For this review, take the finished solid that the model builds, in its own axes (mm). Round coordinates to 2 decimals unless told otherwise and drop trailing zeros. Order: outer loops, then holes, each group sorted by start corner. A loop starts at its lowest first (then second) coordinate and runs counter-clockwise, first axis right, second up. Notation, with made-up numbers: (70, 29.5) - (93, 29.5) arc R27 ccw to (93, 48.5) - close; hole circle Ø9 at (-26, -15). An arc over 180 degrees is marked (long way). One line per item, written item: value.
```python
from build123d import *

# Parameters (mm, degrees)
SKETCH1_W                                           = 50.8
SKETCH1_H                                           = 381
BASE_EXTRUDE_DEPTH                                  = 12.7
CSK_FOR_1_4_FLAT_HEAD_MACHINE_SCREW_100_D           = 6.7564
CSK_FOR_1_4_FLAT_HEAD_MACHINE_SCREW_100_CSINK_D     = 12.8778
CSK_FOR_1_4_FLAT_HEAD_MACHINE_SCREW_100_CSINK_ANGLE = 100
FILLET1_R                                           = 6.35
FILLET2_R                                           = 3.048


with BuildPart() as part:
    # Sketch1 → Base-Extrude (new body)
    with BuildSketch(Plane.XY):
        Rectangle(SKETCH1_W, SKETCH1_H)
    extrude(amount=BASE_EXTRUDE_DEPTH)

    # CSK for 1/4 Flat Head Machine Screw (100)1 (through all)
    with Locations(Plane.XY.offset(12.7)):
        with Locations((0, 165.1), (0, -165.1)):
            CounterSinkHole(CSK_FOR_1_4_FLAT_HEAD_MACHINE_SCREW_100_D / 2, CSK_FOR_1_4_FLAT_HEAD_MACHINE_SCREW_100_CSINK_D / 2, counter_sink_angle=CSK_FOR_1_4_FLAT_HEAD_MACHINE_SCREW_100_CSINK_ANGLE)

    # Fillet1
    fillet1_edges = [part.edges().sort_by_distance(p)[0] for p in [
        (25.4, -190.5, 6.35),
        (-25.4, -190.5, 6.35),
        (-25.4, 190.5, 6.35),
        (25.4, 190.5, 6.35),
    ]]
    fillet(fillet1_edges, radius=FILLET1_R)

    # Fillet2
    fillet2_edges = [part.edges().sort_by_distance(p)[0] for p in [
        (25.4, 0, 12.7),
        (0, -190.5, 12.7),
        (0, 190.5, 12.7),
        (-25.4, 0, 12.7),
        (23.540128061, 188.640128061, 12.7),
        (-23.540128061, 188.640128061, 12.7),
        (-23.540128061, -188.640128061, 12.7),
        (23.540128061, -188.640128061, 12.7),
    ]]
    fillet(fillet2_edges, radius=FILLET2_R)


solid = part.part
```
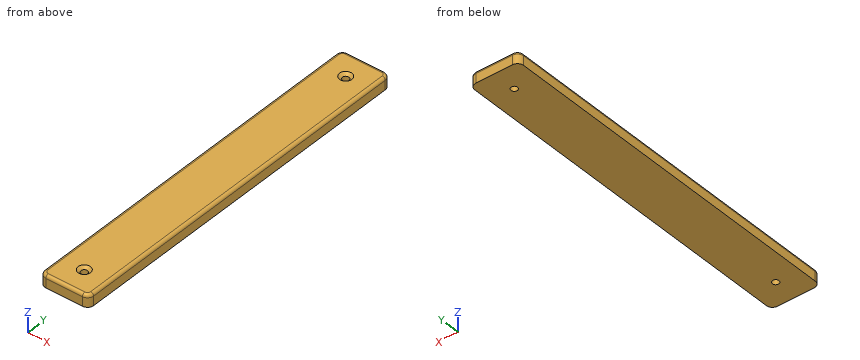
Item 1: Take a section at A-A (y = -165.1). Write out the cut boundary in (x, z).
Returned:
outline: (-25.4, 0) - (-3.38, 0) - (-3.38, 10.13) - (-6.44, 12.7) - (-22.35, 12.7) arc R3.05 ccw to (-25.4, 9.65) - close; (3.38, 0) - (25.4, 0) - (25.4, 9.65) arc R3.05 ccw to (22.35, 12.7) - (6.44, 12.7) - (3.38, 10.13) - close
Item 2: Take a section at B-B (x = 0). Write out the cut boundary in (y, z), plus the area to 3 significant figures.
Returned:
outline: (-190.5, 0) - (-168.48, 0) - (-168.48, 10.13) - (-171.54, 12.7) - (-187.45, 12.7) arc R3.05 ccw to (-190.5, 9.65) - close; (-161.72, 0) - (161.72, 0) - (161.72, 10.13) - (158.66, 12.7) - (-158.66, 12.7) - (-161.72, 10.13) - close; (168.48, 0) - (190.5, 0) - (190.5, 9.65) arc R3.05 ccw to (187.45, 12.7) - (171.54, 12.7) - (168.48, 10.13) - close
area: 4,650 mm^2
Item 3: Wall thickness on line 1 (Y direction, x = 0, z = 5); line 2 (X direction, y = 165.1, z = 2.75); line 3 (Y direction, x = 1.5, z = 12): over which ranges is each line inside the solid? List them lowest first.
Returned:
line 1: -190.5 to -168.48, -161.72 to 161.72, 168.48 to 190.5
line 2: -25.4 to -3.38, 3.38 to 25.4
line 3: -189.4 to -170.5, -159.7 to 159.7, 170.5 to 189.4
